```python
from build123d import *

# Parameters (mm, degrees)
F1_DEPTH = 30
F2_W     = 2.5
F2_H     = 6.7
F3_DEPTH = 17
F4_R     = 1.3
F5_DEPTH = 10.001


with BuildPart() as f1:
    # F0 (on Right) → F1 (new body)
    with BuildSketch(Plane.YZ):
        with BuildLine():
            Line((-11.2, 0), (-11.2, -13.2))
            Line((-11.2, -13.2), (11.2, -13.2))
            Line((11.2, -13.2), (11.2, 0))
            ThreePointArc((11.2, 0), (0, -11.2), (-11.2, 0))
        make_face()
    extrude(amount=F1_DEPTH)

    # F2 (on face) → F3 (join)
    with BuildSketch(Plane(origin=(0, 0, -13.2), x_dir=(1, 0, 0), z_dir=(0, 0, -1))):
        with Locations((8.75, 7.85)):
            Rectangle(F2_W, F2_H)
        with Locations((8.75, -7.85)):
            Rectangle(F2_W, F2_H)
    extrude(amount=-F3_DEPTH)

    # F4 (on face) → F5 (cut, through all)
    with BuildSketch(Plane.YZ.offset(10)):
        with Locations((-7.85, -0.45)):
            Circle(F4_R)
        with Locations((7.85, -0.45)):
            Circle(F4_R)
    extrude(amount=-F5_DEPTH, mode=Mode.SUBTRACT)


solid = f1.part
```
Verification items for the finished model (mm, model axes). A direction names the side the tool comes from. Round coordinates to 2 decimals unless told otherwise and drop trailing zeros. Write each loop counter-clockwise with the first axis right and the second up, starting at its lowest first coordinate (ties: lowest second). Pieces come first, ordered by that corner, then holes. Notation, with made-up numbers: (46, 81) -> (51, 81) arc R24 cw to (51, 96) -> close; hole circle Ø3 at (-19, 61.5). An arc over 180 degrees is marked (long way). Write each question's results on one line, items separated by ' | '. Start each with the question number.
1. Cross-section at C-C (z = -1.25). Enter the section's corners in (x, y).
2. Set-up check for faces 1 (the flat face through (9, -8, 3.8)), 2 (the flat face through (10, -7, -2)), 3 (the flat face through (9, 4.5, -3)), 4 (the flat face through (7.5, 7, -2)), 5 (the flat face through (15, -11.2, -6)): record each of +Z, -Z, +X, -X, +Y, -Y from which the full face is reachable in a straight line by a thin tool's end or side.
3. Cross-section at D-D (x = 21.5). Enter the section's corners in (y, z).
4. Cross-section at A-A (z = -7). Enter the section's corners in (x, y).
5. Draft check along Y on faces 6 (the flat face through (15, 11.2, -7)), 7 (the flat face through (30, -0.1, -11.5)), 8 (the cylindrical face through (14.8, 0.2, -11.2)). Enter one of: +Y half, -Y half, draft (parallel to the pull), parting line (faces both ways), or undercut.
6. Cross-section at B-B (y = 7.85). Enter the section's corners in (x, z).
7. Depth check by flat-ended pin: P1, Ø7.5, axis at y = -7, z = -4.5, coming from the +X side; P2, Ø4, axis at x = 23, y = -6.5, coming from the +Z side; P3, Ø1.5, axis at x = 4.5, y = -1.5, coming from the +Z side; P4, Ø2, axis at y = 9, z = -1.5, coming from the +X side. Enter the tip coordinate at first touch or a pass-through.
8. Material ranges on probe 1 along Z at (x, y) = (9.05, -7.85); probe 2 along X at (y, z) = (4.75, 1); probe 3 along Y at (x, z) = (23.25, -8), recorded low to high. Write a range as from..to.
Solutions:
1) outline: (0, -11.2) -> (30, -11.2) -> (30, -11.13) -> (10, -11.13) -> (10, -8.87) -> (7.5, -8.87) -> (7.5, -11.13) -> (0, -11.13) -> close; (0, 11.13) -> (7.5, 11.13) -> (7.5, 8.87) -> (10, 8.87) -> (10, 11.13) -> (30, 11.13) -> (30, 11.2) -> (0, 11.2) -> close; (7.5, -6.83) -> (10, -6.83) -> (10, -4.5) -> (7.5, -4.5) -> close; (7.5, 4.5) -> (10, 4.5) -> (10, 6.83) -> (7.5, 6.83) -> close
2) face 1: +Z, +X, -X, +Y, -Y | face 2: +Z, +X | face 3: +Z, +X, -X | face 4: +Z, -X | face 5: +Z, -Z, +X, -X, -Y
3) outline: (-11.2, -13.2) -> (11.2, -13.2) -> (11.2, 0) arc R11.2 cw to (-11.2, 0) -> close
4) outline: (0, -11.2) -> (30, -11.2) -> (30, -8.74) -> (10, -8.74) -> (10, -4.5) -> (7.5, -4.5) -> (7.5, -8.74) -> (0, -8.74) -> close; (0, 8.74) -> (7.5, 8.74) -> (7.5, 4.5) -> (10, 4.5) -> (10, 8.74) -> (30, 8.74) -> (30, 11.2) -> (0, 11.2) -> close
5) face 6: +Y half | face 7: draft | face 8: undercut
6) outline: (0, -13.2) -> (30, -13.2) -> (30, -7.99) -> (10, -7.99) -> (10, -1.75) -> (7.5, -1.75) -> (7.5, -7.99) -> (0, -7.99) -> close; (7.5, 0.85) -> (10, 0.85) -> (10, 3.8) -> (7.5, 3.8) -> close
7) P1: stops at x = 30 | P2: stops at z = -7.29 | P3: stops at z = -10.97 | P4: stops at x = 10
8) probe 1: z = -13.2..-1.75, 0.85..3.8 | probe 2: x = 7.5..10 | probe 3: y = -11.2..-7.84, 7.84..11.2
